Design review of the part built by this model. Coordinates are the model's own, in mm. A direction names the side the tool comes from. Give positions to 0.01 mm unless a question says otherwise; leave off trailing zeros. Loops run counter-clockwise (first coordinate to the right, second up) from the corner with the lowest first, then second, coordinate; pieces in that order, holes last. Notation, with made-up numbers: M -24,-12 L 1,-12 A29 ccw 1,12 Z; hole C 49,80 d11. An arc over 180 degrees is marked long. Answer as CSV lines item,"result".
```python
from build123d import *

# Parameters (mm, degrees)
F1_DEPTH = 10
F2_R     = 1.5
F3_DEPTH = 25


with BuildPart() as f1:
    # F0 (on Right) → F1 (new body)
    with BuildSketch(Plane.YZ):
        Polygon((20, 0), (0, 0), (0, -7), (2, -7), (2, -2), (20, -2), align=None)
    extrude(amount=F1_DEPTH)

    # F2 (on face) → F3 (cut)
    with BuildSketch(Plane.XY):
        with Locations((5, 16)):
            Circle(F2_R)
        with Locations((5, 11)):
            Circle(F2_R)
    extrude(amount=-F3_DEPTH, mode=Mode.SUBTRACT)


solid = f1.part
```
1. We need section B-B, the plane z = -1.5. Write out the cut boundary in (x, y), plus the area to 3 significant figures.
Answer block:
outline,"M 0,0 L 10,0 L 10,20 L 0,20 Z; hole C 5,11 d3; hole C 5,16 d3"
area,"186 mm²"
2. We need section D-D, the plane z = -3.75. Write out the cut boundary in (x, y).
Answer block:
outline,"M 0,0 L 10,0 L 10,2 L 0,2 Z"
3. We need section A-A, the plane y = 11. Write out the cut boundary in (x, z), plus the area to 3 significant figures.
Answer block:
outline,"M 0,-2 L 3.5,-2 L 3.5,0 L 0,0 Z; M 6.5,-2 L 10,-2 L 10,0 L 6.5,0 Z"
area,"14.0 mm²"
4. The part is to be moulded in two halves that separate along X. For faces 3 (the flat face through (10, 8, -1)), 4 (the cylindrical face through (6.386, 10.425, -0.986)), 5 (the flat face through (5, 1, -7)), say which applies: pulls with the +X half, pulls with the -X half, needs draft (parallel to the pull), parting line crosses it, or undercut.
Answer block:
face 3,"pulls with the +X half"
face 4,"undercut"
face 5,"needs draft"
5. To check wall thickness, follow L1, parallel to Y at x = 5, z = -0.8; L2, parallel to Y at x = 8.5, z = -2.5; L3, parallel to Z at x = 3, y = 4.5. State the ranges of each line that lie inside material, in increasing order. Write a range as [from, to].
Answer block:
L1,"[0, 9.5], [12.5, 14.5], [17.5, 20]"
L2,"[0, 2]"
L3,"[-2, 0]"
6. For faces 1 (the flat face through (5, 9, -2)), 2 (the flat face through (5, 8, 0)), list the 3-axis set-ups (+Z, -Z, +X, -X, +Y, -Y) from which the entire face can be reached by the end or side of a thin tool; tool diameter is ignored.
Answer block:
face 1,"-Z, +X, -X, +Y"
face 2,"+Z, +X, -X, +Y, -Y"
7. We need section C-C, the plane x = 5. Write out the cut boundary in (y, z), plus the area to 3 significant figures.
Answer block:
outline,"M 0,-7 L 2,-7 L 2,-2 L 9.5,-2 L 9.5,0 L 0,0 Z; M 12.5,-2 L 14.5,-2 L 14.5,0 L 12.5,0 Z; M 17.5,-2 L 20,-2 L 20,0 L 17.5,0 Z"
area,"38.0 mm²"
8. For P1, Ø1.5, axis at x = 6, z = -6, coming from the +Y side, flat-tipped, find the tip position at first contact; note if it passes through.
Answer block:
P1,"y = 2"
